Work out the finished part from the listing and answer in its coordinate system (mm). A direction names the side the tool comes from. Round coordinates to 2 decimals unless told otherwise and drop trailing zeros. Loops run counter-clockwise (first coordinate to the right, second up) from the corner with the lowest first, then second, coordinate; pieces in that order, holes last.
```python
from build123d import *

# Parameters (mm, degrees)
F1_W     = 80
F1_H     = 78.6831277681
F1_R     = 12.7
F2_DEPTH = 25.4
F3_T     = -2.54


with BuildPart() as f2:
    # F1 (on face) → F2 (new body)
    with BuildSketch(Plane.XY):
        Rectangle(F1_W, F1_H)
        Circle(F1_R, mode=Mode.SUBTRACT)
    extrude(amount=F2_DEPTH)

    # F3
    f3_openings = [f2.faces().sort_by_distance(p)[0] for p in [
        (38.877902, 0, 25.4),
    ]]
    offset(amount=F3_T, openings=f3_openings)


solid = f2.part
```
1. Which of the six approach directions +Z, -Z, +X, -X, +Y, -Y give full straight-line access (tool end or side, diameter ignored) to faces 1 (the face through (-40, -1, 13)), 2 (the face through (-12.094, -9.273, 13.81))?
Answer key:
face 1: +Z, -Z, -X, +Y, -Y
face 2: +Z
2. Consider probe 1 along Y at (x, z) = (0, 15.5); probe 2 along Y at (x, z) = (-31.5, 14.25); probe 3 along X at (y, z) = (20, 10.5). Determine where each line is inside the solid, lowest interval first.
Answer key:
probe 1: y = -39.34 to -36.8, -15.24 to -12.7, 12.7 to 15.24, 36.8 to 39.34
probe 2: y = -39.34 to -36.8, 36.8 to 39.34
probe 3: x = -40 to -37.46, 37.46 to 40
3. Find section C-C (y = 0). Write down the section's boundary in (x, z), then the cut area to 3 significant figures.
Answer key:
outline: (-40, 0) - (-12.7, 0) - (-12.7, 25.4) - (-15.24, 25.4) - (-15.24, 2.54) - (-37.46, 2.54) - (-37.46, 25.4) - (-40, 25.4) - close; (12.7, 0) - (40, 0) - (40, 25.4) - (37.46, 25.4) - (37.46, 2.54) - (15.24, 2.54) - (15.24, 25.4) - (12.7, 25.4) - close
area: 371 mm2
4. Find section B-B (x = 0). Write down the section's boundary in (y, z), then the cut area to 3 significant figures.
Answer key:
outline: (-39.34, 0) - (-12.7, 0) - (-12.7, 25.4) - (-15.24, 25.4) - (-15.24, 2.54) - (-36.8, 2.54) - (-36.8, 25.4) - (-39.34, 25.4) - close; (12.7, 0) - (39.34, 0) - (39.34, 25.4) - (36.8, 25.4) - (36.8, 2.54) - (15.24, 2.54) - (15.24, 25.4) - (12.7, 25.4) - close
area: 368 mm2
5. Find section D-D (x = -20). Write down the section's boundary in (y, z), then the cut area to 3 significant figures.
Answer key:
outline: (-39.34, 0) - (39.34, 0) - (39.34, 25.4) - (36.8, 25.4) - (36.8, 2.54) - (-36.8, 2.54) - (-36.8, 25.4) - (-39.34, 25.4) - close
area: 316 mm2
6. Find section A-A (z = 13.5). Write down the section's boundary in (x, y), then the cut area to 3 significant figures.
Answer key:
outline: (-40, -39.34) - (40, -39.34) - (40, 39.34) - (-40, 39.34) - close; circle Ø30.48 at (0, 0); hole (-37.46, -36.8) - (37.46, -36.8) - (37.46, 36.8) - (-37.46, 36.8) - close; hole circle Ø25.4 at (0, 0)
area: 1,000 mm2
7. Determine the mould class of faces 3 (the face through (-1, 17, 2.54)), 4 (the face through (-1, -39.342, 13)), 5 (the face through (-3.5, 12.5, 25.4)), 6 (the face through (37.46, -1, 14)) for opening direction Y: +Y half, -Y half, draft (parallel to the pull), parting line (faces both ways), or undercut.
Answer key:
face 3: undercut
face 4: -Y half
face 5: draft
face 6: undercut
